Check sheet for the modelled part. Datum: model origin and axes. Units: mm. Face numbers are marked on the shaded views. Round coordinates to 2 decimals unless told otherwise and drop trailing zeros. Write each loop counter-clockwise with the first axis right and the second up, starting at its lowest first coordinate (ties: lowest second). Pieces come first, ordered by that corner, then holes. Notation, with made-up numbers: M -31.75,78.5 L 0.25,78.5 A26 cw 0.25,100.5 Z; hole C 82.25,76 d5. An arc over 180 degrees is marked long. Answer in a Markdown table with one row per item.
```python
from build123d import *

# Parameters (mm, degrees)
SKETCH1_R           = 10.00125
BOSS_EXTRUDE1_DEPTH = 203.2
SKETCH2_R           = 10.00125
BOSS_EXTRUDE2_DEPTH = 25.7175
SKETCH4_R           = 3.048
CUT_EXTRUDE1_DEPTH  = 25.4
CHAMFER1_SIZE       = 0.508


with BuildPart() as part:
    # Sketch1 → Boss-Extrude1 (new body)
    with BuildSketch(Plane(origin=(0, 0, 0), x_dir=(1, 0, 0), z_dir=(0, 1, 0))):
        Circle(SKETCH1_R)
    extrude(amount=BOSS_EXTRUDE1_DEPTH)

    # Sketch2 → Boss-Extrude2 (add)
    with BuildSketch(Plane(origin=(0, 203.2, 0), x_dir=(1, 0, 0), z_dir=(0, 1, 0))):
        Circle(SKETCH2_R)
    extrude(amount=BOSS_EXTRUDE2_DEPTH)

    # Sketch4 → Cut-Extrude1 (cut)
    with BuildSketch(Plane(origin=(10.00125, 0, 0), x_dir=(0, 0, -1), z_dir=(1, 0, 0))):
        with Locations((0, 220.0275)):
            Circle(SKETCH4_R)
    extrude(amount=-CUT_EXTRUDE1_DEPTH, mode=Mode.SUBTRACT)

    # Chamfer1
    chamfer1_edges = [part.edges().sort_by_distance(p)[0] for p in [
        (-10.00125, 228.9175, 0),
    ]]
    chamfer(chamfer1_edges, length=CHAMFER1_SIZE)


solid = part.part
```
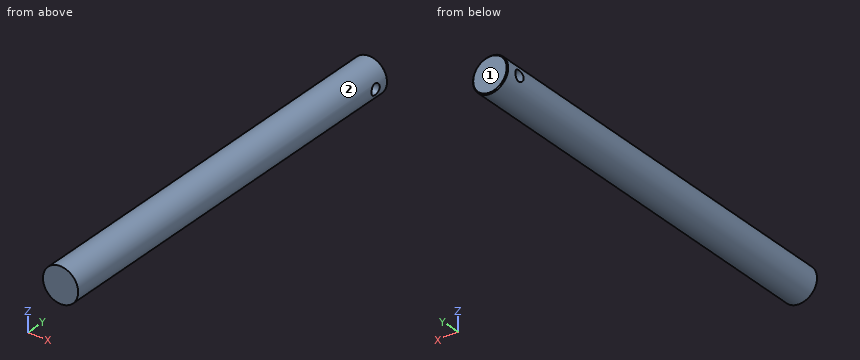
1. Section check B-B, the plane y = 214. Record the cut outline in (x, z).
Found:
| item | result |
|---|---|
| outline | C 0,0 d20 |
2. Scan lines: L1, parallel to Y at x = 1, z = 0; L2, parallel to Y at x = 0.5, z = -0.75; L3, parallel to Z at x = 0.5, y = 53. Record each from-to range of solid material in increasing order.
Found:
| item | result |
|---|---|
| L1 | y = 0 to 216.98, 223.08 to 228.92 |
| L2 | y = 0 to 217.07, 222.98 to 228.92 |
| L3 | z = -9.99 to 9.99 |
3. Draft check along X on the marked faces 1 and 2. Enter one of: +X half, -X half, draft (parallel to the pull), parting line (faces both ways), or undercut.
Found:
| item | result |
|---|---|
| face 1 | draft |
| face 2 | parting line |
4. Go/stop test with flat-tipped pins: pin 1 (4 mm diameter, centred on x = -7, y = 110, fed in from -Z); pin 2 (4 mm diameter, centred on x = 6, y = 46.5, fed in from -Z); pin 3 (2 mm diameter, centred on y = 202.5, z = 7, fed in from -X); pin 4 (5.5 mm diameter, centred on y = 220.03, z = 0, fed in from -X). Record where each tip stops, or that it passes through.
Found:
| item | result |
|---|---|
| pin 1 | stops at z = -8.66 |
| pin 2 | stops at z = -9.17 |
| pin 3 | stops at x = -8 |
| pin 4 | passes through |
5. Section check A-A, the plane z = 0. Record the cut outline in (x, y), and give its area (3 significant figures).
Found:
| item | result |
|---|---|
| outline | M -10,0 L 10,0 L 10,216.98 L -10,216.98 Z; M -10,223.08 L 10,223.08 L 10,228.41 L 9.49,228.92 L -9.49,228.92 L -10,228.41 Z |
| area | 4,460 mm2 |
